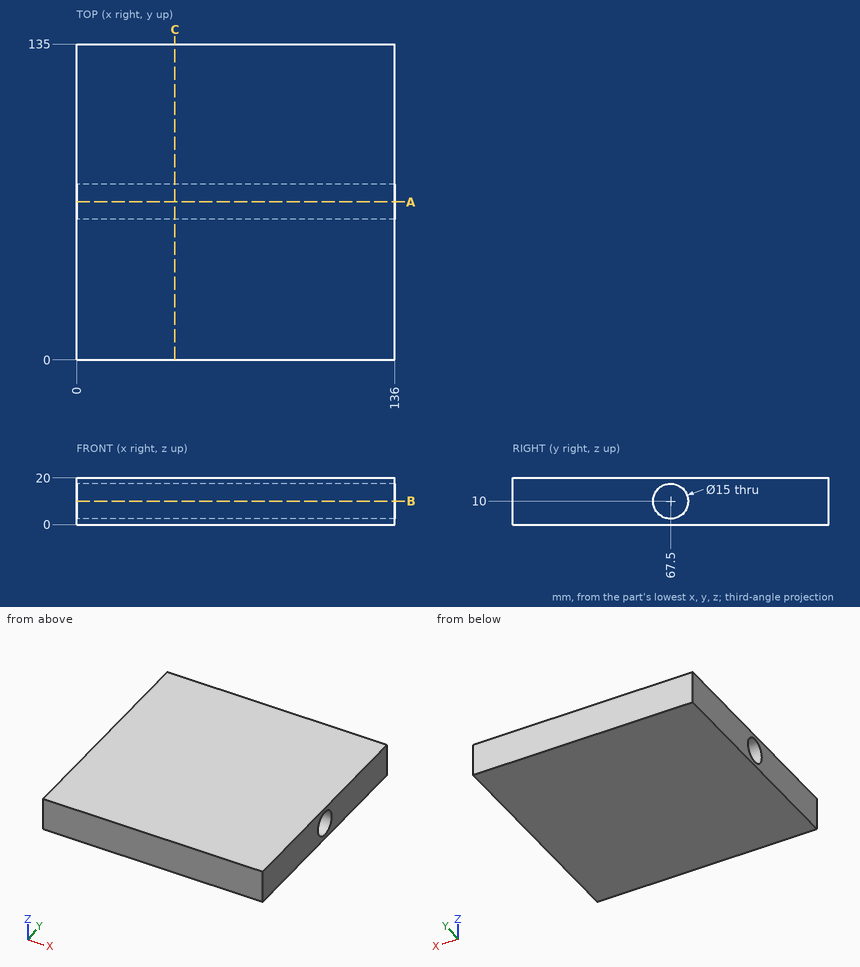
Answer from the drawing. Dimensions are ordinates in mm from the lowest x, y and z of the part. Coordinates: 2 decimals unless noted, no trailing zeros. Write each loop counter-clockwise with the first axis right and the second up, starting at its lowest first coordinate (ties: lowest second). Pieces come first, ordered by that corner, then holes. Notation, with made-up numbers: M -15,1.5 L 24,1.5 A22 ccw 24,33.5 Z; hole C -2.75,74 d8. An arc over 180 degrees is marked long. Write item = value, one per line.
1. The part is cut by section A-A (y = 67.5). Determine the outline of the cut face in (x, z).
Solution:
outline = M 0,0 L 136,0 L 136,2.5 L 0,2.5 Z; M 0,17.5 L 136,17.5 L 136,20 L 0,20 Z
2. Straight lines are drawn through the part: line 1 (Z direction, x = 35, y = 67); line 2 (Y direction, x = 95, z = 11.5); line 3 (Y direction, x = 114, z = 13.5). For each, find the intervals that lie inside material, in ascending order. Write a range as from..to.
Solution:
line_1 = 0..2.52, 17.48..20
line_2 = 0..60.15, 74.85..135
line_3 = 0..60.87, 74.13..135
3. The part is cut by section B-B (z = 10). Determine the outline of the cut face in (x, y), then the cut area to 3 significant figures.
Solution:
outline = M 0,0 L 136,0 L 136,60 L 0,60 Z; M 0,75 L 136,75 L 136,135 L 0,135 Z
area = 16,300 mm2
4. The part is cut by section C-C (x = 42). Determine the outline of the cut face in (y, z), then the cut area to 3 significant figures.
Solution:
outline = M 0,0 L 135,0 L 135,20 L 0,20 Z; hole C 67.5,10 d15
area = 2,520 mm2
